```python
from build123d import *

# Parameters (mm, degrees)
SKETCH1_R           = 20
BOSS_EXTRUDE1_DEPTH = 10
CAVITY3_START       = 0.1
CAVITY3_DEPTH       = 9.9
CUT_EXTRUDE1_DEPTH  = 11
CIRPATTERN1_COUNT   = 11
SKETCH3_R           = 2.75
CUT_EXTRUDE2_DEPTH  = 11
SKETCH4_R           = 4.803689075
CUT_EXTRUDE3_DEPTH  = 6


# Read off the part's stored shape, not the designer's step: Cavity3
with BuildPart() as part:
    # Sketch1 → Boss-Extrude1 (new body)
    with BuildSketch(Plane.XY):
        Circle(SKETCH1_R)
    extrude(amount=BOSS_EXTRUDE1_DEPTH)

    # Cavity3 outline → Cavity3 (cut)
    with BuildSketch(Plane.XY.offset(CAVITY3_START)):
        with BuildLine():
            Line((-19.657828248, -3.683719394), (-12.793623997, 4.45))
            Line((-12.793623997, 4.45), (-12.793623997, 4.95))
            Line((-12.793623997, 4.95), (-19.377757868, 4.95))
            ThreePointArc((-19.377757868, 4.95), (-19.989485324, 0.648441592), (-19.657828248, -3.683719394))
        make_face()
    extrude(amount=CAVITY3_DEPTH, mode=Mode.SUBTRACT)

    # Sketch2 → Cut-Extrude1 (cut)
    with BuildSketch(Plane.XY.offset(10)):
        Polygon((-18.893600606, -4.32866599), (-20.741181365, -6.51795158), (-20.741181365, 5.95), (-19.377757868, 5.95), (-11.793623997, 5.95), (-11.793623997, 4.084431193), align=None)
    cut_extrude1 = extrude(amount=-CUT_EXTRUDE1_DEPTH, mode=Mode.SUBTRACT)

    # CirPattern1: Cut-Extrude1 ×11 about axis
    cirpattern1_axis = Axis((0, 0, 0), (0, 0, 1))
    for i in range(1, CIRPATTERN1_COUNT):
        add(cut_extrude1.rotate(cirpattern1_axis, i * 360 / CIRPATTERN1_COUNT), mode=Mode.SUBTRACT)

    # Sketch3 → Cut-Extrude2 (cut)
    with BuildSketch(Plane(origin=(0, 0, 0), x_dir=(-1, 0, 0), z_dir=(0, 0, -1))):
        Circle(SKETCH3_R)
    extrude(amount=-CUT_EXTRUDE2_DEPTH, mode=Mode.SUBTRACT)

    # Sketch4 → Cut-Extrude3 (cut)
    with BuildSketch(Plane(origin=(0, 0, 0), x_dir=(-1, 0, 0), z_dir=(0, 0, -1))):
        Circle(SKETCH4_R)
    extrude(amount=-CUT_EXTRUDE3_DEPTH, mode=Mode.SUBTRACT)


solid = part.part
```
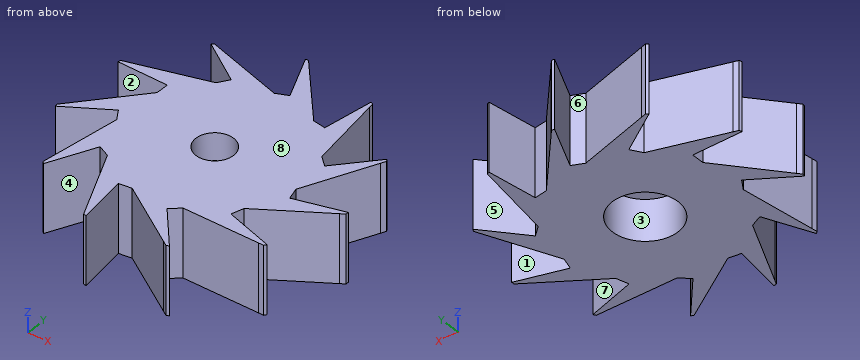
For this review, take the finished solid that the model builds, in its own axes (mm). Face numbers are marked on the shaded views. A direction names the side the tool comes from. Round coordinates to 2 decimals unless told otherwise and drop trailing zeros. Write each loop counter-clockwise with the first axis right and the second up, starting at its lowest first coordinate (ties: lowest second). Pieces come first, ordered by that corner, then holes. Notation, with made-up numbers: (26.5, 28) - (57.5, 28) arc R20 ccw to (57.5, 57) - close; hole circle Ø4 at (69.25, 20.25). An arc over 180 degrees is marked (long way). Put each result on its own line as item: value.
Q1. We need section B-B (x = 0). Give the boundary of the cut face in (y, z), and give its area (3 significant figures).
Solved:
outline: (-13.73, 0) - (-4.8, 0) - (-4.8, 6) - (-2.75, 6) - (-2.75, 10) - (-13.73, 10) - close; (2.75, 6) - (4.8, 6) - (4.8, 0) - (12.97, 0) - (12.97, 10) - (2.75, 10) - close; (14.32, 0) - (17.52, 0) - (17.52, 10) - (14.32, 10) - close
area: 219 mm2
Q2. Mouldability with a two-part tool opening along X and no side actions: class the marked faces 6, 7 and 8 as released by +X, released by -X, zero draft, split by the parting line, or undercut.
Solved:
face 6: undercut
face 7: released by +X
face 8: zero draft
Q3. We need section C-C (x = 11.5). Give the boundary of the cut face in (y, z), and give its area (3 significant figures).
Solved:
outline: (-11.5, 0) - (-9.58, 0) - (-9.58, 10) - (-11.5, 10) - close; (-6.36, 0) - (5.64, 0) - (5.64, 10) - (-6.36, 10) - close
area: 139 mm2
Q4. Insertion check: pin 1 Ø3 at (y, z) = (3, 8) entering from -X; pin 2 Ø6.5 at (x, y) = (0, 0) entering from -Z; pin 3 Ø2 at (x, z) = (-6.5, 7) entering from -Y. Each pin has a flat end and moves straight along its axis. Give the tip position at first contact, or say it passes through.
Solved:
pin 1: stops at x = -13.97
pin 2: stops at z = 6
pin 3: stops at y = -15.62
Q5. Machinability: for the marked faces 1, 2, 3, 4 and 5, which of the approach directions +Z, -Z, +X, -X, +Y, -Y give a long, thin tool a straight path to every point of the face, cutting with its end or side? Answer none if there is none.
Solved:
face 1: +Z, -Z
face 2: +Z, -Z, -X
face 3: -Z
face 4: +Z, -Z, -Y
face 5: +Z, -Z, +Y
Q6. We need section A-A (x = -16). Give the boundary of the cut face in (y, z).
Solved:
outline: (-3.21, 0) - (-0.9, 0) - (-0.9, 10) - (-3.21, 10) - close; (5.95, 0) - (7.26, 0) - (7.26, 10) - (5.95, 10) - close
Q7. Wall thickness on probe 1 along Y at (x, z) = (15, 6.75); probe 2 along Y at (x, z) = (0, 7.2); probe 3 along Z at (x, y) = (0, 3.5): over which ranges is each line inside the solid? List them lowest first.
Solved:
probe 1: y = -11.45 to -10.61, -4.04 to -1.8, 5.15 to 8.23
probe 2: y = -13.73 to -2.75, 2.75 to 12.97, 14.32 to 17.52
probe 3: z = 6 to 10
